```python
from build123d import *

# Parameters (mm, degrees)
PAD_DEPTH       = 10
SKETCH001_W     = 25
SKETCH001_H     = 50
POCKET_DEPTH    = 5
SKETCH002_R     = 2
POCKET001_DEPTH = 12
FILLET_R        = 2
FILLET001_R     = 1
POCKET002_DEPTH = 5
SKETCH004_W     = 40
SKETCH004_H     = 30
POCKET003_DEPTH = 5
FILLET002_R     = 1
FILLET003_R     = 1


with BuildPart() as part:
    # Sketch → Pad (new body)
    with BuildSketch(Plane.XY):
        with BuildLine():
            Line((-25, 0), (0, 0))
            Line((0, 0), (0, 40))
            Line((0, 40), (-75, 40))
            Line((-75, 40), (-75, 35))
            Line((-75, 35), (-67, 35))
            Line((-67, 35), (-67, 15))
            Line((-67, 15), (-75, 15))
            Line((-75, 15), (-75, 10))
            add(Edge.make_bspline(
                [(-25, 0), (-25, 10), (-75, 10)],
                knots=[0, 0, 0, 1, 1, 1], degree=2))
        make_face()
    extrude(amount=PAD_DEPTH)

    # Sketch001 → Pocket (cut)
    with BuildSketch(Plane.XY):
        with Locations((-7.5, 20)):
            Rectangle(SKETCH001_W, SKETCH001_H)
    extrude(amount=POCKET_DEPTH, mode=Mode.SUBTRACT)

    # Sketch002 → Pocket001 (cut)
    with BuildSketch(Plane.XY):
        with Locations((-8, 30)):
            Circle(SKETCH002_R)
        with Locations((-8, 10)):
            Circle(SKETCH002_R)
    extrude(amount=POCKET001_DEPTH, mode=Mode.SUBTRACT)

    # Fillet
    fillet_edges = [part.edges().sort_by_distance(p)[0] for p in [
        (0, 40, 7.5),
        (0, 0, 7.5),
        (-75, 10, 5),
        (-75, 40, 5),
    ]]
    fillet(fillet_edges, radius=FILLET_R)

    # Fillet001
    fillet001_edges = [part.edges().sort_by_distance(p)[0] for p in [
        (-25, 0, 5),
    ]]
    fillet(fillet001_edges, radius=FILLET001_R)

    # Sketch003 (on Face13 of Fillet001) → Pocket002 (cut)
    with BuildSketch(Plane(origin=(0, 40, 0), x_dir=(-1, 0, 0), z_dir=(0, 1, 0))):
        Polygon((62, -5), (62, 5), (59, 5), (59, 15), (54, 15), (54, 5), (51, 5), (51, -5), align=None)
        Polygon((46, -5), (46, 5), (43, 5), (43, 15), (38, 15), (38, 5), (35, 5), (35, -5), align=None)
    extrude(amount=-POCKET002_DEPTH, mode=Mode.SUBTRACT)

    # Sketch004 (on Face5 of Pocket002) → Pocket003 (cut)
    with BuildSketch(Plane(origin=(0, 0, 0), x_dir=(1, 0, 0), z_dir=(0, 0, -1))):
        with Locations((-40, -15)):
            Rectangle(SKETCH004_W, SKETCH004_H)
    extrude(amount=-POCKET003_DEPTH, mode=Mode.SUBTRACT)

    # Fillet002
    fillet002_edges = [part.edges().sort_by_distance(p)[0] for p in [
        (-62, 37.5, 5),
        (-59, 37.5, 5),
        (-46, 37.5, 5),
        (-43, 37.5, 5),
        (-43, 37.5, 10),
        (-59, 37.5, 10),
        (-54, 37.5, 5),
        (-38, 37.5, 5),
        (-35, 37.5, 5),
        (-51, 37.5, 5),
        (-54, 37.5, 10),
        (-38, 37.5, 10),
    ]]
    fillet(fillet002_edges, radius=FILLET002_R)

    # Fillet003
    fillet003_edges = [part.edges().sort_by_distance(p)[0] for p in [
        (-35, 37.5, 0),
        (-46, 37.5, 0),
        (-51, 37.5, 0),
        (-62, 37.5, 0),
    ]]
    fillet(fillet003_edges, radius=FILLET003_R)


solid = part.part
```
CAD build for the part. Positions are in the model's coordinates, mm. A direction names the side the tool comes from. Coordinates: 2 decimals unless noted, no trailing zeros. Write each loop counter-clockwise with the first axis right and the second up, starting at its lowest first coordinate (ties: lowest second). Pieces come first, ordered by that corner, then holes. Notation, with made-up numbers: (-19, -14) -> (37, -14) arc R24 ccw to (37, 0) -> close; hole circle Ø10 at (71.25, -2.75). An arc over 180 degrees is marked (long way). Use CSV: the item, a comma, the result in double quotes. Start each with the question number.
Item 1: Wall check: probe 1 along Y at (x, z) = (-8, 7.6); probe 2 along X at (y, z) = (30, 6.45); probe 3 along X at (y, z) = (19, 5.5). Give the ranges that are in metal, low to high.
Item 2: Two-plate mould, pull along X, no slides. Class faces 5 (the cylindrical face through (-0.6, 0.57, 7.54)), 6 (the cylindrical face through (-9.474, 11.352, 7.465)), 7 (the flat face through (-30, 20, 10)): +X half, -X half, draft (parallel to the pull), parting line (faces both ways), or undercut.
Item 3: Band-saw the part on A-A, the plane x = -8. Write the cut outline in (y, z), plus the area to 3 significant figures.
Item 4: Band-saw the part on C-C, the plane x = -23. Write the cut outline in (y, z).
Item 5: Drop flat-ended pins along their axis: P1, Ø4, axis at x = -62, z = 6, coming from the -Y side; P2, Ø6, axis at y = 29.5, z = 7.5, coming from the -X side; P3, Ø1.1, axis at x = -52.5, y = 38.5, coming from the -Z side; P4, Ø3.5, axis at y = 38.5, z = 7, coming from the +X side. Give the stop position or say it passes through.
Item 6: Band-saw the part on D-D, the plane y = 37. Give the number of separate pieces and of enclosed holes in the cut face, plus the area to 3 significant figures.
Item 7: Tool access for faces 1 (the flat face through (-60, 20, 2)), 2 (the flat face through (-43, 38, 7)), 3 (the flat face through (-51, 38, 3)), 4 (the flat face through (-71, 15, 5)): list every direction of +Z, -Z, +X, -X, +Y, -Y with a clear straight run to the whole face (end or side of a thin tool).
Item 8: Band-saw the part on B-B, the plane y = 22. Write the cut outline in (x, z), plus the area to 3 significant figures.
Response values:
1,probe 1,"y = 0 to 8, 12 to 28, 32 to 40"
1,probe 2,"x = -67 to -10, -6 to 0"
1,probe 3,"x = -67 to 0"
2,face 5,"+X half"
2,face 6,"undercut"
2,face 7,"draft"
3,outline,"(0, 5) -> (8, 5) -> (8, 10) -> (0, 10) -> close; (12, 5) -> (28, 5) -> (28, 10) -> (12, 10) -> close; (32, 5) -> (40, 5) -> (40, 10) -> (32, 10) -> close"
3,area,"160 mm2"
4,outline,"(0, 5) -> (30, 5) -> (30, 0) -> (40, 0) -> (40, 10) -> (0, 10) -> close"
5,P1,"stops at y = 9.73"
5,P2,"stops at x = -67"
5,P3,"stops at z = 5"
5,P4,"stops at x = 0"
6,separate pieces,"3"
6,enclosed holes,"0"
6,area,"488 mm2"
7,face 1,"-Z, +X, -Y"
7,face 2,"+Z, -Z, +Y"
7,face 3,"-Z, +Y"
7,face 4,"+Z, -Z, -X"
8,outline,"(-67, 0) -> (-60, 0) -> (-60, 5) -> (0, 5) -> (0, 10) -> (-67, 10) -> close"
8,area,"370 mm2"
